```python
from build123d import *

# Parameters (mm, degrees)
SKETCH_R  = 2.25
PAD_DEPTH = 400
FILLET_R  = 1.5


with BuildPart() as part:
    # Sketch → Pad (new body)
    with BuildSketch(Plane(origin=(0, 0, 0), x_dir=(1, 0, 0), z_dir=(0, 0, -1))):
        Polygon((7, 0), (7, -1), (4, -1), (4, -2.5), (6.499998, -5), (13.500002, -5), (16, -2.5), (16, -1), (13, -1), (13, 0), (20, 0), (20, -7), (19, -7), (19, -4), (17.5, -4), (15.000002, -6.5), (15.000002, -13.500005), (17.5, -16.000005), (19, -16.000005), (19, -13.000005), (20, -13.000005), (20, -20.000005), (13, -20.000005), (13, -19.000005), (16, -19.000005), (16, -17.500005), (13.500002, -15.000005), (6.499998, -15.000005), (4, -17.500005), (4, -19.000005), (7, -19.000005), (7, -20.000005), (0, -20.000005), (0, -13.000005), (1, -13.000005), (1, -16.000005), (2.5, -16.000005), (4.999998, -13.500005), (4.999998, -6.5), (2.5, -4), (1, -4), (1, -7), (0, -7), (0, 0), align=None)
        with Locations((10, -10.000002)):
            Circle(SKETCH_R, mode=Mode.SUBTRACT)
    extrude(amount=PAD_DEPTH)

    # Fillet
    fillet_edges = [part.edges().sort_by_distance(p)[0] for p in [
        (20, 20.000005, -200),
        (20, 0, -200),
        (0, 20.000005, -200),
        (0, 0, -200),
    ]]
    fillet(fillet_edges, radius=FILLET_R)


solid = part.part
```
Can you work these out from the model? Positions are in its coordinate system, mm. A direction names the side the tool comes from. Round coordinates to 2 decimals unless told otherwise and drop trailing zeros. One line per item, written item: value. Start each with the question number.
1. For pin 1 (1.1 mm diameter, centred on x = 0.5, z = -296, fed in from -Y), with a flat end and sliding along its axis, tell me the tip position at first contact or that it passes through.
2. If I drill on probe 1 along X at (y, z) = (14.5, -120.5); probe 2 along Y at (x, z) = (10, -108), over which ranges is the centre line in solid material (lowest first)?
3. For faces 1 (the flat face through (12.4, 9.9, -400)), 2 (the flat face through (10, 5, -197)), which set-ups out of +Z, -Z, +X, -X, +Y, -Y let a thin tool reach every point of the face, with its end or its side?
4. If we mould it in two halves opening along Y, with no side actions, what happens to faces 3 (the flat face through (12.4, 9.9, 0)), 4 (the flat face through (15, 10, -197))? For each: pulls with the +Y half, pulls with the -Y half, needs draft (parallel to the pull), parting line crosses it, or undercut.
Calculated:
1. pin 1: stops at y = 0.07
2. probe 1: x = 0 to 1, 4 to 16, 19 to 20
2. probe 2: y = 5 to 7.75, 12.25 to 15
3. face 1: -Z, +X, -X, +Y, -Y
3. face 2: +Z, -Z
4. face 3: needs draft
4. face 4: undercut
